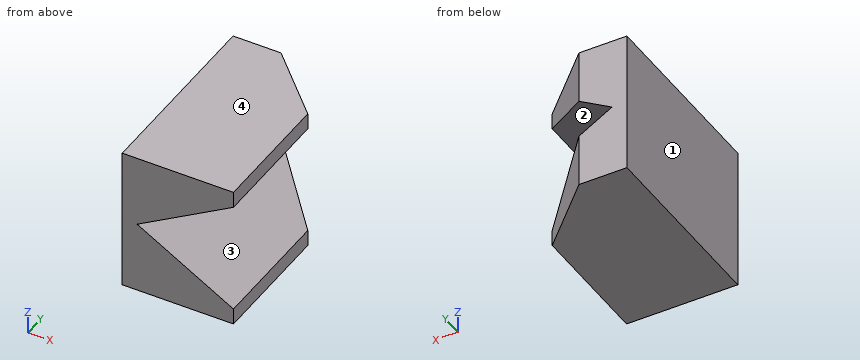
```python
from build123d import *

# Parameters (mm, degrees)
BOSS_EXTRUDE1_DEPTH     = 76.2
CUT_EXTRUDE1_DEPTH      = 95.715964076
CUT_EXTRUDE1_DEPTH_BACK = 95.715964076


with BuildPart() as part:
    # Sketch1 → Boss-Extrude1 (new body)
    with BuildSketch(Plane(origin=(0, 0, 0), x_dir=(1, 0, 0), z_dir=(0, 1, 0))):
        Polygon((44.177534378, 22.321573291), (0, 22.321573291), (0, -34.828426709), (44.177534378, -34.828426709), (44.177534378, -28.342193898), (5.91866733, -6.253426709), (44.177534378, 15.83534048), align=None)
    extrude(amount=BOSS_EXTRUDE1_DEPTH)

    # Sketch3 → Cut-Extrude1 (cut, two sides: drawn at the far end of the back side and taken through both)
    with BuildSketch(Plane.XY.offset(-CUT_EXTRUDE1_DEPTH_BACK)):
        Polygon((-101.492059558, 196.742059558), (19.05, 76.2), (44.177534378, 51.072465622), (164.719593936, -69.469593936), (405.803713052, 171.61452518), (139.592059558, 437.826178674), align=None)
    extrude(amount=CUT_EXTRUDE1_DEPTH + CUT_EXTRUDE1_DEPTH_BACK, mode=Mode.SUBTRACT)


solid = part.part
```
Check sheet for the modelled part. Datum: model origin and axes. Units: mm. Face numbers are marked on the shaded views. Round coordinates to 2 decimals unless told otherwise and drop trailing zeros. Order: outer loops, then holes, each group sorted by start corner. A loop starts at its lowest first (then second) coordinate and runs counter-clockwise, first axis right, second up. Notation, with made-up numbers: (24.25, -21.5) -> (73.25, -21.5) arc R4 ccw to (73.25, -17.5) -> close; hole circle Ø8 at (-11.75, -31.5). An arc over 180 degrees is marked (long way). One line per item, written item: value. Start each with the question number.
Q1. Cross-section at B-B (y = 40). Record the boundary of the cut face in (x, z), and give its area (3 significant figures).
Q2. Mould release check, pull along Z, two halves, no side actions. Record for the marked faces 1, 2, 3 and 4: pulls with the +Z half, pulls with the -Z half, needs draft (parallel to the pull), parting line crosses it, or undercut.
Q3. Cross-section at C-C (x = 16.5). Record the boundary of the cut face in (y, z), and give its area (3 significant figures).
Q4. Gauge pin test, flat ends, axial feed: pin 1 Ø6 at (x, z) = (39.5, -12) entering from +Y; pin 2 Ø4 at (y, z) = (67, -9) entering from +X. Record the tip position at first contact, or that the pin passes through.
Q5. Thickness scan on line 1 (Z direction, x = 22, y = 50); line 2 (Z direction, x = 27.5, y = 45); line 3 (X direction, y = 6, z = -15). Record the ranges inside material, lowest first.
Q6. Cross-section at A-A (x = 24.5). Record the boundary of the cut face in (y, z), and give its area (3 significant figures).
Q7. Cross-section at D-D (z = 19.5). Record the boundary of the cut face in (x, y).
Completed:
1. outline: (0, -22.32) -> (44.18, -22.32) -> (44.18, -15.84) -> (5.92, 6.25) -> (44.18, 28.34) -> (44.18, 34.83) -> (0, 34.83) -> close
1. area: 1,680 mm²
2. face 1: needs draft
2. face 2: undercut
2. face 3: undercut
2. face 4: pulls with the +Z half
3. outline: (0, -22.32) -> (76.2, -22.32) -> (76.2, 0.14) -> (0, 0.14) -> close; (0, 12.36) -> (76.2, 12.36) -> (76.2, 34.83) -> (0, 34.83) -> close
3. area: 3,420 mm²
4. pin 1: stops at y = 58.75
4. pin 2: stops at x = 30.25
5. line 1: z = -22.32 to -3.03, 15.54 to 34.83
5. line 2: z = -22.32 to -6.21, 18.71 to 34.83
5. line 3: x = 0 to 42.73
6. outline: (0, -22.32) -> (70.75, -22.32) -> (70.75, -4.47) -> (0, -4.47) -> close; (0, 16.98) -> (70.75, 16.98) -> (70.75, 34.83) -> (0, 34.83) -> close
6. area: 2,530 mm²
7. outline: (0, 0) -> (28.86, 0) -> (28.86, 66.39) -> (19.05, 76.2) -> (0, 76.2) -> close
